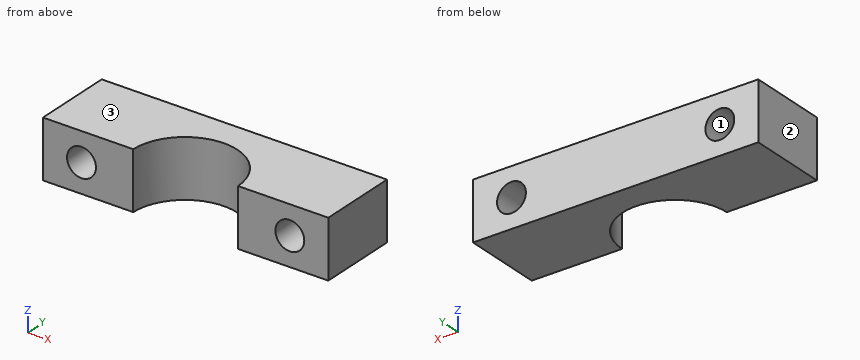
Autodesk Inventor part; units mm, degrees
ref_plane "Work Plane1" through (-18.034, -15.556, -6) normal (0, 0, -1) x (0, 1, 0)
ref_plane "YZ Plane" through (0, 0, 0) normal (1, 0, 0) x (0, 1, 0)
ref_plane "XZ Plane" through (0, 0, 0) normal (0, 1, 0) x (-1, 0, 0)
sketch "Sketch1" plane through (0, 0, 0) normal (0, 0, 1) x (1, 0, 0)
  line L0 (-14.8291, -4.1038) -> (-14.8291, 4.1962)
  line L1 (-14.8291, -4.1038) -> (-5.4491, -4.1038)
  arc A0 (5.4491, -4.1038) -> (-5.4491, -4.1038) centre (0, -4.2038) ccw
  line L2 (5.4491, -4.1038) -> (14.8291, -4.1038)
  line L3 (14.8291, -4.1038) -> (14.8291, 4.1962)
  line L4 (-14.8291, 4.1962) -> (14.8291, 4.1962)
ref_plane "Work Plane1" through (-18.034, -15.556, -6) normal (0, 0, -1) x (0, 1, 0)
extrude "Extrusion1" add sketch "Sketch1" against normal up to surface (6 mm away)
sketch "Sketch2" plane through (-14.8291, 4.1962, 0) normal (0, 1, 0) x (1, 0, 0)
  circle A0 centre (4, 3) radius 1.5
  circle A1 centre (25.6582, 3) radius 1.5
  point P0 (14.8291, 0)
extrude "Extrusion2" cut sketch "Sketch2" against normal through all
properties part number "pylon_actuator_holder_jaw"
For this review, take the finished solid that the model builds, in its own axes (mm). Face numbers are marked on the shaded views. Round coordinates to 2 decimals unless told otherwise and drop trailing zeros. Write each loop counter-clockwise with the first axis right and the second up, starting at its lowest first coordinate (ties: lowest second). Pieces come first, ordered by that corner, then holes. Notation, with made-up numbers: (13, -33.75) - (20, -33.75) arc R20 cw to (20, -15.75) - close; hole circle Ø11 at (-13, 40). An arc over 180 degrees is marked (long way). Answer as a JSON object with one key per item and string values.
1. We need section A-A on y = -0.5. Give the boundary of the cut face in (x, z), then the cut area to 3 significant figures.
Response values:
{"outline": "(-14.83, -6) - (-4, -6) - (-4, 0) - (-14.83, 0) - close; (4, -6) - (14.83, -6) - (14.83, 0) - (4, 0) - close; hole circle Ø3 at (-10.83, -3); hole circle Ø3 at (10.83, -3)", "area": "116 mm2"}
2. For pin 1 Ø1.5 at (x, y) = (-1, -0.5) entering from +Z, flat-tipped, find the tip position at first contact; note if it passes through.
Response values:
{"pin 1": "passes through"}
3. Draft analysis for pull direction Z (two halves, no side actions). For the marked faces 1, 2 and 3, state which applies: +Z half, -Z half, draft (parallel to the pull), parting line (faces both ways), or undercut.
Response values:
{"face 1": "undercut", "face 2": "draft", "face 3": "+Z half"}
4. We need section D-D on y = -2.75. Give the boundary of the cut face in (x, z).
Response values:
{"outline": "(-14.83, -6) - (-5.25, -6) - (-5.25, 0) - (-14.83, 0) - close; (5.25, -6) - (14.83, -6) - (14.83, 0) - (5.25, 0) - close; hole circle Ø3 at (-10.83, -3); hole circle Ø3 at (10.83, -3)"}
5. We need section C-C on z = -5.45. Give the boundary of the cut face in (x, y).
Response values:
{"outline": "(-14.83, -4.1) - (-5.45, -4.1) arc R5.45 cw to (5.45, -4.1) - (14.83, -4.1) - (14.83, 4.2) - (-14.83, 4.2) - close"}
6. To check wall thickness, follow line 1 along X through (y, z) = (-0.5, -3); line 2 along X through (y, z) = (3.5, -4.1); line 3 along Z through (x, y) = (-10.5, 1.25). State the ranges of each line that lie inside material, in increasing order.
Response values:
{"line 1": "x = -14.83 to -12.33, -9.33 to -4, 4 to 9.33, 12.33 to 14.83", "line 2": "x = -14.83 to -11.85, -9.81 to 9.81, 11.85 to 14.83", "line 3": "z = -6 to -4.46, -1.54 to 0"}
7. We need section B-B on z = -3. Give the boundary of the cut face in (x, y).
Response values:
{"outline": "(-14.83, -4.1) - (-12.33, -4.1) - (-12.33, 4.2) - (-14.83, 4.2) - close; (-9.33, -4.1) - (-5.45, -4.1) arc R5.45 cw to (5.45, -4.1) - (9.33, -4.1) - (9.33, 4.2) - (-9.33, 4.2) - close; (12.33, -4.1) - (14.83, -4.1) - (14.83, 4.2) - (12.33, 4.2) - close"}
